```python
from build123d import *

# Parameters (mm, degrees)
F0_R     = 3.175
F0_R_2   = 1.5872946887
F1_DEPTH = 3.048


with BuildPart() as f1:
    # F0 (on Front) → F1 (new body)
    with BuildSketch(Plane.XZ):
        with BuildLine():
            ThreePointArc((-9.0974841174, 95.7674032941), (-9.0871801878, 96.0230192533), (-9.0837447185, 96.2788197363))
            ThreePointArc((-9.0837447185, 96.2788197363), (-18.4042625744, 105.801624578), (-28.124965097, 96.6876897734))
            ThreePointArc((-28.124965097, 96.6876897734), (-19.0688946406, 86.764941082), (-9.0974841174, 95.7674032941))
        make_face()
        with Locations((-18.6087447185, 96.2788197363)):
            Circle(F0_R, mode=Mode.SUBTRACT)
        with BuildLine():
            ThreePointArc((-9.0974841174, 95.7674032941), (-19.0688946406, 86.764941082), (-28.124965097, 96.6876897734))
            Line((-28.124965097, 96.6876897734), (-34.0306231002, 49.2433344929))
            ThreePointArc((-34.0306231002, 49.2433344929), (-17.7281897242, 61.3293971023), (-2.8642383786, 47.5125525358))
            Line((-2.8642383786, 47.5125525358), (-9.0974841174, 95.7674032941))
        make_face()
        with Locations((-20.5585247247, 82.0040197363)):
            Circle(F0_R_2, mode=Mode.SUBTRACT)
        with BuildLine():
            Line((-34.4828878032, 45.6099701438), (-34.0306231002, 49.2433344929))
            ThreePointArc((-34.0306231002, 49.2433344929), (-34.3618557694, 47.4397347289), (-34.4828878032, 45.6099701438))
        make_face()
        with BuildLine():
            ThreePointArc((-2.8642383786, 47.5125525358), (-17.7281897242, 61.3293971023), (-34.0306231002, 49.2433344929))
            Line((-34.0306231002, 49.2433344929), (-34.4828878032, 45.6099701438))
            Line((-34.4828878032, 45.6099701438), (-34.376407934, 43.6385798228))
            ThreePointArc((-34.376407934, 43.6385798228), (-19.5826293255, 29.6337397487), (-3.1846463922, 41.7208232156))
            Line((-3.1846463922, 41.7208232156), (-2.7533729136, 44.6833300781))
            ThreePointArc((-2.7533729136, 44.6833300781), (-2.7384161803, 45.0809499292), (-2.7334295582, 45.4788197363))
            ThreePointArc((-2.7334295582, 45.4788197363), (-2.7661655158, 46.4977873569), (-2.8642383786, 47.5125525358))
        make_face()
        with Locations((-18.6084295582, 45.4788197363)):
            Circle(F0_R, mode=Mode.SUBTRACT)
        with BuildLine():
            Line((-2.6184752397, 45.6099701438), (-2.8642383786, 47.5125525358))
            ThreePointArc((-2.8642383786, 47.5125525358), (-2.7661655158, 46.4977873569), (-2.7334295582, 45.4788197363))
            ThreePointArc((-2.7334295582, 45.4788197363), (-2.7384161803, 45.0809499292), (-2.7533729136, 44.6833300781))
            Line((-2.7533729136, 44.6833300781), (-2.6184752397, 45.6099701438))
        make_face()
        with BuildLine():
            Line((-34.376407934, 43.6385798228), (-34.4828878032, 45.6099701438))
            ThreePointArc((-34.4828878032, 45.6099701438), (-34.4603235704, 44.6226181096), (-34.376407934, 43.6385798228))
        make_face()
        with BuildLine():
            ThreePointArc((-3.1846463922, 41.7208232156), (-19.5826293255, 29.6337397487), (-34.376407934, 43.6385798228))
            Line((-34.376407934, 43.6385798228), (-31.0182580763, -18.5349012397))
            ThreePointArc((-31.0182580763, -18.5349012397), (-21.7640756728, -8.4996467927), (-11.9821216689, -18.0211802637))
            ThreePointArc((-11.9821216689, -18.0211802637), (-14.5569871682, -24.5343404354), (-20.8894718888, -27.5261333803))
            Line((-20.8894718888, -27.5261333803), (22.9428783311, -25.9586802637))
            ThreePointArc((22.9428783311, -25.9586802637), (15.0053783311, -18.0211802637), (22.9428783311, -10.0836802637))
            Line((22.9428783311, -10.0836802637), (-1.9724256736, -7.5720420447))
            ThreePointArc((-1.9724256736, -7.5720420447), (-7.4415456853, -4.5544233197), (-9.0423034299, 1.4833636188))
            Line((-9.0423034299, 1.4833636188), (-3.1846463922, 41.7208232156))
        make_face()
        with BuildLine():
            ThreePointArc((-3.1846463922, 41.7208232156), (-2.899019426, 43.191887665), (-2.7533729136, 44.6833300781))
            Line((-2.7533729136, 44.6833300781), (-3.1846463922, 41.7208232156))
        make_face()
        with BuildLine():
            ThreePointArc((-11.9821216689, -18.0211802637), (-21.7640756728, -8.4996467927), (-31.0182580763, -18.5349012397))
            ThreePointArc((-31.0182580763, -18.5349012397), (-28.0353179292, -24.957193426), (-21.4442641508, -27.5459728563))
            Line((-21.4442641508, -27.5459728563), (-20.8894718888, -27.5261333803))
            ThreePointArc((-20.8894718888, -27.5261333803), (-14.5569871682, -24.5343404354), (-11.9821216689, -18.0211802637))
        make_face()
        with Locations((-21.5071216689, -18.0211802637)):
            Circle(F0_R, mode=Mode.SUBTRACT)
        with BuildLine():
            Line((-20.8894718888, -27.5261333803), (-21.4442641508, -27.5459728563))
            ThreePointArc((-21.4442641508, -27.5459728563), (-21.1667234508, -27.540095856), (-20.8894718888, -27.5261333803))
        make_face()
        with BuildLine():
            ThreePointArc((30.8803783311, -18.0211802637), (28.5555384067, -12.408520188), (22.9428783311, -10.0836802637))
            ThreePointArc((22.9428783311, -10.0836802637), (15.0053783311, -18.0211802637), (22.9428783311, -25.9586802637))
            ThreePointArc((22.9428783311, -25.9586802637), (28.5555384067, -23.6338403394), (30.8803783311, -18.0211802637))
        make_face()
        with Locations((22.9428783311, -18.0211802637)):
            Circle(F0_R, mode=Mode.SUBTRACT)
    extrude(amount=F1_DEPTH)


solid = f1.part
```
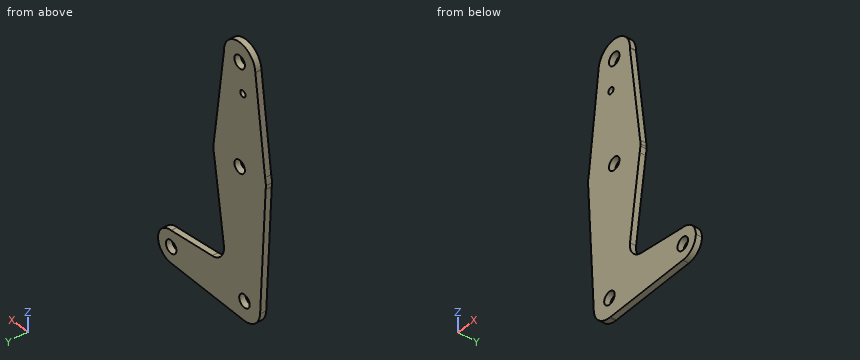
Model file for the job. Use its own axes, mm. Give positions to 0.01 mm unless a question says otherwise; leave off trailing zeros. Write each loop counter-clockwise with the first axis right and the second up, starting at its lowest first coordinate (ties: lowest second). Pieces come first, ordered by that corner, then holes. Notation, with made-up numbers: (25, 11) -> (53, 11) arc R21 cw to (53, 42) -> close; hole circle Ø2 at (82, 36). An arc over 180 degrees is marked (long way). Use CSV: the item, a comma, the result in double quotes. Start each with the question number.
1) Cut at B-B on z = 70. List the corners of the cut face in (x, y).
2) Drill centre lines: L1, parallel to Z at x = -20.5, y = -0.9; L2, parallel to X at y = -1.5, z = 95; L3, parallel to X at y = -0.45, z = 96. Where is each one in solid material? Low to high.
3) Cut at A-A on y = -1.15. Count the separate pieces of the cut face and the enclosed holes in it, plus the area to 3 significant figures.
4) Cut at C-C on x = 7. List the corners of the cut face in (y, z).
5) Pin check, flat tips, straight feed: P1, Ø1, axis at x = 22.5, y = -0.5, coming from the +Z side; P2, Ø1, axis at y = -2, z = 73.5, coming from the -X side; P3, Ø1, axis at x = 8.5, y = -0.5, coming from the -Z side. Stop position of each tip, or through.
Final values:
1,outline,"(-31.45, -3.05) -> (-5.77, -3.05) -> (-5.77, 0) -> (-31.45, 0) -> close"
2,L1,"z = -27.51 to -21.03, -15.01 to 42.93, 48.03 to 80.42, 83.59 to 93.73, 98.83 to 105.61"
2,L2,"x = -28.34 to -21.51, -15.7 to -9"
2,L3,"x = -28.21 to -21.77, -15.45 to -9.09"
3,separate pieces,"1"
3,enclosed holes,"5"
3,area,"3,820 mm2"
4,outline,"(-3.05, -26.53) -> (0, -26.53) -> (0, -8.48) -> (-3.05, -8.48) -> close"
5,P1,"stops at z = -9.99"
5,P2,"stops at x = -31.07"
5,P3,"stops at z = -26.49"
